```python
from build123d import *

# Parameters (mm, degrees)
SKETCH2_W           = 23
SKETCH2_H           = 80
SKETCH2_R           = 10
BOSS_EXTRUDE1_DEPTH = 1
SKETCH3_W           = 80
SKETCH3_H           = 10
SKETCH3_R           = 2.5
BOSS_EXTRUDE2_DEPTH = 1


with BuildPart() as part:
    # Sketch2 → Boss-Extrude1 (new body)
    with BuildSketch(Plane(origin=(0, 0, 0), x_dir=(1, 0, 0), z_dir=(0, 1, 0))):
        Rectangle(SKETCH2_W, SKETCH2_H)
        with Locations(Location((0, 0, 0), (0, 0, 270))):
            Circle(SKETCH2_R, mode=Mode.SUBTRACT)
    extrude(amount=BOSS_EXTRUDE1_DEPTH)

    # Sketch3 → Boss-Extrude2 (add)
    with BuildSketch(Plane.ZY.offset(11.5)):
        with Locations((0, 5)):
            Rectangle(SKETCH3_W, SKETCH3_H)
        with Locations((-25, 6)):
            Circle(SKETCH3_R, mode=Mode.SUBTRACT)
        with Locations(Location((25, 6, 0), (0, 0, 180))):
            Circle(SKETCH3_R, mode=Mode.SUBTRACT)
    boss_extrude2 = extrude(amount=BOSS_EXTRUDE2_DEPTH)

    # Mirror1: Boss-Extrude2 across plane
    add(boss_extrude2.mirror(Plane(origin=(0, 0, 0), x_dir=(0, 0, 1), z_dir=(1, 0, 0))))


solid = part.part
```
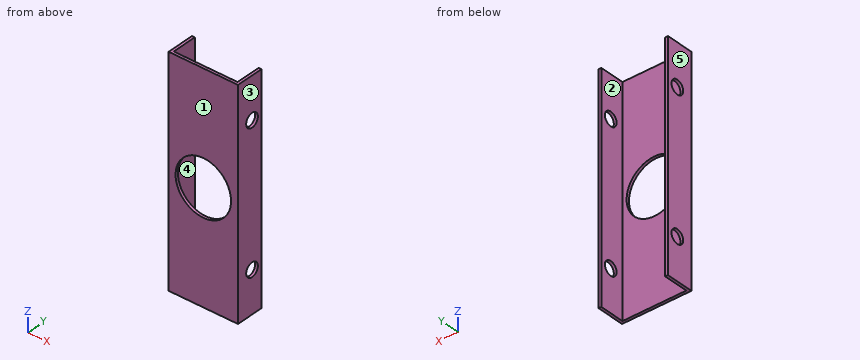
The model under review builds one solid part; all positions refer to its coordinate system, in mm. Face numbers are marked on the shaded views. A direction names the side the tool comes from. Give positions to 0.01 mm unless a question says otherwise; leave off trailing zeros. Loops run counter-clockwise (first coordinate to the right, second up) from the corner with the lowest first, then second, coordinate; pieces in that order, holes last. Notation, with made-up numbers: (70, 9) - (86, 9) arc R17 cw to (86, 26) - close; hole circle Ø5 at (66, -39). An arc over 180 degrees is marked (long way). Answer as a JSON object with one key per item and string values.
Q1. Add section C-C on z = 0. State the section outline as (x, y) points, plus the area to 3 significant figures.
Worked out:
{"outline": "(-12.5, 0) - (-10, 0) - (-10, 1) - (-11.5, 1) - (-11.5, 10) - (-12.5, 10) - close; (10, 0) - (12.5, 0) - (12.5, 10) - (11.5, 10) - (11.5, 1) - (10, 1) - close", "area": "23.0 mm^2"}
Q2. For the marked faces 4 and 5, list the 3-axis set-ups (+Z, -Z, +X, -X, +Y, -Y) from which the entire face can be reached by the end or side of a thin tool; tool diameter is ignored.
Worked out:
{"face 4": "+Z, -Z, +Y", "face 5": "+Z, -Z, -X, +Y, -Y"}
Q3. Add section D-D on y = 1.75. State the section outline as (x, z) points.
Worked out:
{"outline": "(-12.5, -40) - (-11.5, -40) - (-11.5, 40) - (-12.5, 40) - close; (11.5, -40) - (12.5, -40) - (12.5, 40) - (11.5, 40) - close"}
Q4. Insertion check: pin 1 (6 mm diameter, centred on x = -2, z = -24, fed in from -Y); pin 2 (4 mm diameter, centred on x = 4, z = 13.5, fed in from +Y). Each pin has a flat end and moves straight along its axis. Give the tip position at first contact, or say it passes through.
Worked out:
{"pin 1": "stops at y = 0", "pin 2": "stops at y = 1"}
Q5. To check wall thickness, follow line 1 along X through (y, z) = (8, 3); line 2 along Y through (x, z) = (7.5, -8); line 3 along Y through (x, z) = (11.85, -25). State the ranges of each line that lie inside material, in increasing order.
Worked out:
{"line 1": "x = -12.5 to -11.5, 11.5 to 12.5", "line 2": "y = 0 to 1", "line 3": "y = 0 to 3.5, 8.5 to 10"}
Q6. Add section B-B on x = 0. State the section outline as (y, z) points.
Worked out:
{"outline": "(0, -40) - (1, -40) - (1, -10) - (0, -10) - close; (0, 10) - (1, 10) - (1, 40) - (0, 40) - close"}
Q7. Add section A-A on y = 6. State the section outline as (x, z) points.
Worked out:
{"outline": "(-12.5, -40) - (-11.5, -40) - (-11.5, -27.5) - (-12.5, -27.5) - close; (-12.5, -22.5) - (-11.5, -22.5) - (-11.5, 22.5) - (-12.5, 22.5) - close; (-12.5, 27.5) - (-11.5, 27.5) - (-11.5, 40) - (-12.5, 40) - close; (11.5, -40) - (12.5, -40) - (12.5, -27.5) - (11.5, -27.5) - close; (11.5, -22.5) - (12.5, -22.5) - (12.5, 22.5) - (11.5, 22.5) - close; (11.5, 27.5) - (12.5, 27.5) - (12.5, 40) - (11.5, 40) - close"}
Q8. Mouldability with a two-part tool opening along X and no side actions: class the marked faces 1, 2 and 3 as +X half, -X half, draft (parallel to the pull), parting line (faces both ways), or undercut.
Worked out:
{"face 1": "draft", "face 2": "undercut", "face 3": "+X half"}
